Can you work these out from the model? Positions are in its coordinate system, mm. A direction names the side the tool comes from. Round coordinates to 2 decimals unless told otherwise and drop trailing zeros. Loops run counter-clockwise (first coordinate to the right, second up) from the corner with the lowest first, then second, coordinate; pieces in that order, holes last.
Autodesk Inventor part; units mm, degrees
ref_plane "YZ Plane" through (0, 0, 0) normal (1, 0, 0) x (0, 1, 0)
ref_plane "XZ Plane" through (0, 0, 0) normal (0, 1, 0) x (-1, 0, 0)
ref_plane "XY Plane" through (0, 0, 0) normal (0, 0, 1) x (1, 0, 0)
ref_plane "Work Plane1" through (55, -70.0761, -12.5) normal (1, 0, 0) x (0, 0, -1)
ref_plane "Work Plane2" through (-33.6954, 10.9239, 2.7231) normal (0, 0, 1) x (1, 0, 0)
sketch "Sketch2" plane through (-33.6954, 10.9239, 2.7231) normal (0, 0, 1) x (1, 0, 0)
  line L0 (-55, -33.4239) -> (0, -33.4239)
  line L1 (0, -33.4239) -> (0, 11.5761)
  line L2 (0, 11.5761) -> (-55, 11.5761)
  line L3 (-55, 11.5761) -> (-55, -33.4239)
  line L4 (-55, 1.5761) -> (-41, 1.5761)
  line L5 (-41, 1.5761) -> (-41, 11.5761)
  line L6 (-7.5, -26.9239) -> (-7.5, -33.4239)
  line L7 (-7.5, 5.0761) -> (-7.5, 11.5761)
  line L8 (-7.5, -26.9239) -> (0, -26.9239)
  line L9 (-47.5, -10.9239) -> (-55, -10.9239)
  point P0 (-27.5, 11.5761)
  dimension "d4" = 55
  dimension "d5" = 45
  dimension "d10" = 14
  dimension "d11" = 10
  dimension "d14" = 40
  dimension "d15" = 32
  dimension "d23" = 16
extrude "Extrusion1" add sketch "Sketch2" along normal blind 7 contours L3 L4 L5 L2 L1 L8 L6 L0 | L6 L8 L1 L0
hole "Hole1" at (-41.1954, -16, 2.7231) at (-41.1954, 16, 2.7231) at (-81.1954, 0, 2.7231) direction (0, 0, 1) diameter 6 end through all
fillet "Fillet1" radius 2 6 edges at (-81.6954, 12.5, 9.7231) (-88.6954, -5, 9.7231) (-74.6954, 17.5, 9.7231) (-54.1954, 22.5, 9.7231) (-61.1954, -22.5, 9.7231) (-33.6954, 0, 9.7231)
properties part number "Print-head_Mount"
(1) If we section it at C-C, the plane y = 0: List the corners of the cut face in (x, z) for me, then the cut area to 3 significant figures.
Worked answers:
outline: (-88.7, 2.72) - (-84.2, 2.72) - (-84.2, 9.72) - (-86.7, 9.72) arc R2 ccw to (-88.7, 7.72) - close; (-78.2, 2.72) - (-33.7, 2.72) - (-33.7, 7.72) arc R2 ccw to (-35.7, 9.72) - (-78.2, 9.72) - close
area: 341 mm2
(2) If I drill on line 1 (X direction, y = -16, z = 7.5); line 2 (X direction, y = 0, z = 5.5); line 3 (Y direction, x = -39, z = 8.75), over which ranges is the centre line in solid material (lowest first)?
Worked answers:
line 1: x = -88.7 to -44.2, -38.2 to -33.7
line 2: x = -88.7 to -84.2, -78.2 to -33.7
line 3: y = -22.22 to -18.04, -13.96 to 13.96, 18.04 to 22.22
(3) Will this pin go through, and if not, where does the flat tip stop? P1, Ø4, axis at x = -78.5, z = 5, coming from the +Y side.
Worked answers:
P1: stops at y = 12.5
(4) If we section it at A-A, the plane y = 16: List the corners of the cut face in (x, z) for me.
Worked answers:
outline: (-74.7, 2.72) - (-44.2, 2.72) - (-44.2, 9.72) - (-72.7, 9.72) arc R2 ccw to (-74.7, 7.72) - close; (-38.2, 2.72) - (-33.7, 2.72) - (-33.7, 7.72) arc R2 ccw to (-35.7, 9.72) - (-38.2, 9.72) - close
(5) If we mould it in two halves opening along X, with no side actions, what happens to faces 4 (the cylindrical face through (-43.223, -18.211, 6.272)), 5 (the cylindrical face through (-74.125, 16.584, 9.122)), 6 (the cylindrical face through (-43.223, 13.789, 6.272)), 7 (the flat face through (-62, -22.5, 5))? For each: released by +X, released by -X, zero draft, split by the parting line, or undercut.
Worked answers:
face 4: undercut
face 5: released by -X
face 6: undercut
face 7: zero draft
(6) For faces 1 (the cylindrical face through (-84.17, -0.39, 6.27)), 2 (the cylindrical face through (-80.58, 11.93, 9.12)), 3 (the flat face through (-82, 12.5, 5)), which set-ups out of +Z, -Z, +X, -X, +Y, -Y let a thin tool reach every point of the face, with its end or its side?
Worked answers:
face 1: +Z, -Z
face 2: +Z, -X, +Y
face 3: +Z, -Z, -X, +Y
(7) If we section it at B-B, the plane z = 6.75: List the corners of the cut face in (x, y) for me, then the cut area to 3 significant figures.
Worked answers:
outline: (-88.7, -22.5) - (-33.7, -22.5) - (-33.7, 22.5) - (-74.7, 22.5) - (-74.7, 12.5) - (-88.7, 12.5) - close; hole circle Ø6 at (-81.2, 0); hole circle Ø6 at (-41.2, -16); hole circle Ø6 at (-41.2, 16)
area: 2,250 mm2
